Design review of the part built by this model. Coordinates are the model's own, in mm. A direction names the side the tool comes from. Give positions to 0.01 mm unless a question says otherwise; leave off trailing zeros. Order: outer loops, then holes, each group sorted by start corner. A loop starts at its lowest first (then second) coordinate and runs counter-clockwise, first axis right, second up. Notation, with made-up numbers: (4, 50) -> (25, 50) arc R28 cw to (25, 81) -> close; hole circle Ø5 at (-39.5, -18.5). An arc over 180 degrees is marked (long way). One line per item, written item: value. Start each with the question number.
1) Consider section C-C (x = -14.5). State the section outline as (y, z) points (3 decimals).
2) The part is to be moulded in two halves that separate along X. For faces 4 (the face through (-34.52, 8.1, 1.61)), 5 (the face through (-15, 0, 2)), 6 (the face through (-35.4, 16.3, 1.6)), say which applies: released by +X, released by -X, zero draft, split by the parting line, or undercut.
3) Consider section A-A (y = 10.75). State the section outline as (x, z) points (3 decimals).
4) Tool access review of faces 1 (the face through (-11.882, 14.445, 3.551)), 2 (the face through (-11.8, 16.1, 3.6)), 3 (the face through (-11.886, 1.745, 3.551)): name each direction out of +Z, -Z, +X, -X, +Y, -Y from which nothing blocks a thin tool from reaching the whole face with its end or side.
5) For pin 1 (0.8 mm diameter, centred on x = -22.5, z = 3.5, fed in from +Y); pin 2 (1.5 mm diameter, centred on x = -32.5, z = 3, fed in from +Y); pin 3 (8 mm diameter, centred on x = -32.5, y = 7.5, fed in from +Z) (3 decimals), all flat-tipped, find the tip position at first contact; note any pin that passes through.
6) Consider section B-B (z = 2.6). State the section outline as (x, y) points (3 decimals).
7) Wall thickness on line 1 along Y through (x, z) = (-20, 3.5); line 2 along Z through (x, y) = (-25, 8.25) (3 decimals); line 3 along X through (y, z) = (9, 0.4): over which ranges is each line inside the solid? List them lowest first. Write a range as from..to.
from build123d import *

# Parameters (mm, degrees)
F0_W     = 38.1
F0_H     = 19.05
F1_DEPTH = 3.175
F2_R     = 2.3454703993
F3_DEPTH = 3.176
F5_DEPTH = 0.762


with BuildPart() as f1:
    # F0 (on Top) → F1 (new body)
    with BuildSketch(Plane.XY):
        with Locations((-19.05, 9.525)):
            Rectangle(F0_W, F0_H)
    extrude(amount=F1_DEPTH)

    # F2 (on face) → F3 (cut, through all)
    with BuildSketch(Plane.XY.offset(3.175)):
        with Locations((-32.6583981514, 9.525)):
            Circle(F2_R)
        with BuildLine():
            ThreePointArc((-38.1, 9.9683756083), (-35.308362686, 16.3938160997), (-28.8257542998, 19.05))
            Line((-28.8257542998, 19.05), (-38.1, 19.05))
            Line((-38.1, 19.05), (-38.1, 9.9683756083))
        make_face()
        with BuildLine():
            ThreePointArc((-28.8257542998, 0), (-35.308362686, 2.6561839003), (-38.1, 9.0816243917))
            Line((-38.1, 9.0816243917), (-38.1, 0))
            Line((-38.1, 0), (-28.8257542998, 0))
        make_face()
    extrude(amount=-F3_DEPTH, mode=Mode.SUBTRACT)

    # F4 (on face) → F5 (join)
    with BuildSketch(Plane.XY.offset(3.175)):
        with BuildLine():
            add(Edge.make_bspline(
                [(-26.5377387404, 15.9110687673), (-26.7108747115, 15.8254740139), (-26.8840106825, 15.7398792605), (-27.0571466535, 15.654284507)],
                knots=[0, 0, 0, 0, 0.579415858, 0.579415858, 0.579415858, 0.579415858], degree=3))
            Line((-27.0571466535, 15.654284507), (-27.0571466535, 2.7385666035))
            add(Edge.make_bspline(
                [(-27.0571466535, 2.7385666035), (-27.0795693358, 2.6088543631), (-27.1225207817, 2.3603859501), (-26.8266557283, 2.183014384), (-26.6604257883, 2.1276841688), (-26.579702273, 2.1008150652)],
                knots=[0, 0, 0, 0, 0.359730405, 0.6890763936, 1, 1, 1, 1], degree=3))
            Line((-26.579702273, 2.1008150652), (-24.8697847128, 2.1008150652))
            add(Edge.make_bspline(
                [(-24.8697847128, 2.1008150652), (-24.8535585114, 1.9993606342), (-24.820613422, 1.7933712454), (-25.0545304604, 1.6052521128), (-25.323348361, 1.3860952125), (-24.5846096398, 1.4667534331), (-23.7811649583, 1.5054977354), (-22.5648546478, 1.5317740605), (-21.8525212711, 1.4849440744), (-20.7065855211, 1.6821403738), (-19.5728440966, 2.0528020227), (-19.1090591627, 2.3669456633), (-18.9018342644, 2.5073089637)],
                knots=[0, 0, 0, 0, 0.0654142898, 0.1328147962, 0.1852280569, 0.2717986293, 0.3900220534, 0.5225934237, 0.6267763583, 0.7573014589, 0.891559262, 1, 1, 1, 1], degree=3))
            Line((-18.9018342644, 2.5073089637), (-17.4452550709, 2.5073089637))
            add(Edge.make_bspline(
                [(-17.4452550709, 2.5073089637), (-17.416342407, 2.3859721487), (-17.3563210578, 2.1340825495), (-17.0722687387, 2.1058012821), (-16.9250462204, 2.0911432803)],
                knots=[0, 0, 0, 0, 0.4817063324, 1, 1, 1, 1], degree=3))
            Line((-16.9250462204, 2.0911432803), (-14.0298530459, 2.0911432803))
            Line((-14.0298530459, 2.0911432803), (-14.0298530459, 1.0200680699))
            Line((-14.0298530459, 1.0200680699), (-9.6812043339, 2.4914150126))
            add(Edge.make_bspline(
                [(-9.6812043339, 2.4914150126), (-9.6409541279, 2.4226709942), (-9.5613256349, 2.2866721227), (-9.3732923035, 2.143877022), (-9.146753539, 2.1258439034), (-8.9577295904, 2.2565656827), (-8.9125275808, 2.4112662698), (-8.8891088963, 2.4914150126)],
                knots=[0, 0, 0, 0, 0.2053847319, 0.4063203233, 0.6002825129, 0.7929105851, 1, 1, 1, 1], degree=3))
            Line((-8.8891088963, 2.4914150126), (-8.0058202147, 2.4914150126))
            Line((-8.0058202147, 2.4914150126), (-8.0058202147, 2.6511875913))
            Line((-8.0058202147, 2.6511875913), (-8.8891088963, 2.6511875913))
            add(Edge.make_bspline(
                [(-8.8891088963, 2.6511875913), (-8.9310142556, 2.7313268058), (-9.0111442626, 2.8845662941), (-9.2288589733, 2.9502078721), (-9.4263111029, 2.954461386), (-9.5681762791, 2.7983408667), (-9.6258537843, 2.6991547711), (-9.6537470818, 2.6511875913)],
                knots=[0, 0, 0, 0, 0.2243735688, 0.4290395288, 0.619806208, 0.816135277, 1, 1, 1, 1], degree=3))
            Line((-9.6537470818, 2.6511875913), (-13.9779066667, 4.1145463474))
            Line((-13.9779066667, 4.1145463474), (-13.9779066667, 3.2444412354))
            Line((-13.9779066667, 3.2444412354), (-16.2190869451, 3.2444412354))
            Line((-16.2190869451, 3.2444412354), (-16.2190869451, 8.471253328))
            Line((-16.2190869451, 8.471253328), (-12.8844231367, 8.471253328))
            add(Edge.make_bspline(
                [(-12.8844231367, 8.471253328), (-12.4868405129, 8.3912644099), (-11.73186638, 8.2393725502), (-10.9755685718, 7.6600087014), (-10.0278228964, 7.0776029449), (-9.2641156682, 6.3657609783), (-8.4323489729, 5.5191632424), (-8.2256469446, 5.2628506515), (-8.4263613819, 4.9657352945), (-8.4045845677, 4.387056325), (-8.3245215623, 3.8946895211), (-7.8349969225, 3.3357865397), (-7.3142777062, 2.8825893477), (-7.0247473195, 2.6306025684)],
                knots=[0, 0, 0, 0, 0.1119269029, 0.2125392595, 0.3204849305, 0.4302536688, 0.542538281, 0.5958954746, 0.6528186178, 0.7312491143, 0.8038353409, 0.8909284931, 1, 1, 1, 1], degree=3))
            Line((-7.0247473195, 2.6306025684), (-6.4539997838, 3.1442753971))
            Line((-6.4539997838, 3.1442753971), (-5.8452025987, 2.6306025684))
            add(Edge.make_bspline(
                [(-5.8452025987, 2.6306025684), (-5.7510163843, 2.5382953385), (-5.5793479133, 2.3700515982), (-5.3068982698, 2.3599422662), (-5.0234062685, 2.629445519), (-5.1548387797, 2.7849198566), (-5.217380356, 2.8589016292)],
                knots=[0, 0, 0, 0, 0.2794125753, 0.5092712331, 0.7664888973, 1, 1, 1, 1], degree=3))
            Line((-5.217380356, 2.8589016292), (-5.9783770703, 3.4867241047))
            Line((-5.9783770703, 3.4867241047), (-5.217380356, 4.190646112))
            Line((-5.217380356, 4.190646112), (-4.3422332965, 3.5247737542))
            add(Edge.make_bspline(
                [(-4.3422332965, 3.5247737542), (-4.2753552319, 3.4833438946), (-4.1355489457, 3.396736203), (-3.8719087651, 3.5821675688), (-3.8873582518, 3.8259382225), (-3.9635831277, 3.9291369105), (-4.0002227761, 3.9787422866)],
                knots=[0, 0, 0, 0, 0.2503847052, 0.5234205857, 0.7709185888, 1, 1, 1, 1], degree=3))
            Line((-4.0002227761, 3.9787422866), (-4.7757523134, 4.6124062501))
            Line((-4.7757523134, 4.6124062501), (-4.2272070423, 5.1231207326))
            Line((-4.2272070423, 5.1231207326), (-5.0594825298, 5.8891922235))
            add(Edge.make_bspline(
                [(-5.0594825298, 5.8891922235), (-5.2342245953, 6.0119831219), (-5.5535406301, 6.2363658579), (-5.9633037959, 6.3380845337), (-6.4624834448, 6.3629289512), (-6.9588518276, 6.326635918), (-7.2564382113, 6.1799434156), (-7.404985372, 6.1067184433)],
                knots=[0, 0, 0, 0, 0.2203014043, 0.4025691847, 0.6016033984, 0.8011310759, 1, 1, 1, 1], degree=3))
            add(Edge.make_bspline(
                [(-7.404985372, 6.1067184433), (-7.8012870357, 6.5100044394), (-8.5207565636, 7.2421975688), (-9.3143752369, 7.9809513855), (-10.4526059497, 8.667475744), (-11.8318533209, 9.304087771), (-13.1655398172, 9.6100287611), (-13.4780210852, 9.655550231), (-13.5454072432, 9.665475678)],
                knots=[0, 0, 0, 0, 0.1949094928, 0.3542547898, 0.528809926, 0.7243716486, 0.9083314981, 0.9676026394, 0.9676026394, 0.9676026394, 0.9676026394], degree=3))
            Line((-13.5454072432, 9.665475678), (-13.5536914822, 9.665475678))
            Line((-13.5536914822, 9.665475678), (-16.2297561765, 9.665475678))
            Line((-16.2297561765, 9.665475678), (-16.2297561765, 14.7121604532))
            Line((-16.2297561765, 14.7121604532), (-14.0407746658, 14.7121604532))
            Line((-14.0407746658, 14.7121604532), (-14.0407746658, 13.74643296))
            Line((-14.0407746658, 13.74643296), (-9.6628116444, 15.162833035))
            add(Edge.make_bspline(
                [(-9.6628116444, 15.162833035), (-9.5994792917, 15.0419453644), (-9.4666485777, 14.7884096682), (-8.9151551249, 14.924804863), (-8.8862007543, 15.0941198994), (-8.8744670414, 15.162833035)],
                knots=[0, 0, 0, 0, 0.3512906634, 0.7367442472, 1, 1, 1, 1], degree=3))
            Line((-8.8744670414, 15.162833035), (-8.0032702535, 15.162833035))
            Line((-8.0032702535, 15.162833035), (-8.0032702535, 15.3721110607))
            Line((-8.0032702535, 15.3721110607), (-8.8744670414, 15.3721110607))
            add(Edge.make_bspline(
                [(-8.8744670414, 15.3721110607), (-8.9258811293, 15.4535897314), (-9.0257330431, 15.6112970859), (-9.2823856435, 15.7082360182), (-9.5546444314, 15.5282819888), (-9.6134472425, 15.4120218853), (-9.6300745245, 15.3725532584)],
                knots=[0, 0, 0, 0, 0.2589067963, 0.4997338796, 0.7803818448, 0.9274568815, 0.9274568815, 0.9274568815, 0.9274568815], degree=3))
            Line((-9.6300745245, 15.3725532584), (-13.9726913457, 16.8323148205))
            Line((-13.9726913457, 16.8323148205), (-13.9726913457, 15.9259032621))
            Line((-13.9726913457, 15.9259032621), (-17.0669947674, 15.9259032621))
            add(Edge.make_bspline(
                [(-17.0669947674, 15.9259032621), (-17.2379265625, 15.8260077216), (-17.5305453526, 15.6574083814), (-17.5131075408, 15.4495405967), (-17.506107688, 15.3641048819)],
                knots=[0, 0, 0, 0, 0.5880208056, 1, 1, 1, 1], degree=3))
            Line((-17.506107688, 15.3641048819), (-18.9438629895, 15.3641048819))
            add(Edge.make_bspline(
                [(-18.9438629895, 15.3641048819), (-19.0730076064, 15.5122124042), (-19.3699914184, 15.8528037322), (-20.4455895706, 16.0592715534), (-21.1153456714, 16.3460981975), (-21.8142141514, 16.3983614206), (-22.1944451332, 16.4267960936)],
                knots=[0, 0, 0, 0, 0.212159, 0.4878855201, 0.7213756277, 1, 1, 1, 1], degree=3))
            Line((-22.1944451332, 16.4267960936), (-25.1324698329, 16.4267960936))
            add(Edge.make_bspline(
                [(-25.1324698329, 16.4267960936), (-25.0155507598, 16.3238609839), (-24.815014757, 16.1473098455), (-24.822982641, 15.9805868028), (-24.8263049871, 15.9110687673)],
                knots=[0, 0, 0, 0, 0.583032829, 1, 1, 1, 1], degree=3))
            Line((-24.8263049871, 15.9110687673), (-26.5377387404, 15.9110687673))
        make_face()
        with BuildLine():
            Line((-25.8164200932, 3.2712235115), (-25.8011277765, 8.5837785155))
            Line((-25.8011277765, 8.5837785155), (-17.506107688, 8.5837785155))
            Line((-17.506107688, 8.5837785155), (-17.4452550709, 3.1483727507))
            Line((-17.4452550709, 3.1483727507), (-17.4452550709, 2.7118595317))
            Line((-17.4452550709, 2.7118595317), (-18.8643243164, 2.7118595317))
            add(Edge.make_bspline(
                [(-18.8643243164, 2.7118595317), (-19.0815269134, 2.85521998), (-19.5524918726, 3.166071455), (-20.5984014649, 3.5593135264), (-21.5481955341, 3.753304769), (-22.1358927762, 3.7784602355), (-22.4202815443, 3.7906330545)],
                knots=[0, 0, 0, 0, 0.2329927864, 0.5052031588, 0.7605660635, 1, 1, 1, 1], degree=3))
            Line((-22.4202815443, 3.7906330545), (-25.1571703702, 3.7906330545))
            add(Edge.make_bspline(
                [(-25.1571703702, 3.7906330545), (-25.0642022591, 3.6982952356), (-24.8942335308, 3.5294788374), (-24.855211218, 3.3517428953), (-24.837533012, 3.2712235115)],
                knots=[0, 0, 0, 0, 0.5469718577, 1, 1, 1, 1], degree=3))
            Line((-24.837533012, 3.2712235115), (-25.8164200932, 3.2712235115))
        make_face(mode=Mode.SUBTRACT)
        with BuildLine():
            Line((-18.9293026924, 15.1415970176), (-17.506107688, 15.1415970176))
            Line((-17.506107688, 15.1415970176), (-17.428284511, 9.7119892016))
            Line((-17.428284511, 9.7119892016), (-25.822866708, 9.7119892016))
            Line((-25.822866708, 9.7119892016), (-25.822866708, 14.6800291177))
            Line((-25.822866708, 14.6800291177), (-24.7983376545, 14.6800291177))
            add(Edge.make_bspline(
                [(-25.1186843961, 14.1409179196), (-25.0576893253, 14.2285084067), (-24.9435954911, 14.3923500806), (-24.7955780658, 14.5766326071), (-24.7956461395, 14.6560214032), (-24.7983376545, 14.6800291177)],
                knots=[0, 0, 0, 0, 0.4063243511, 0.7600467132, 0.9204385352, 0.9204385352, 0.9204385352, 0.9204385352], degree=3))
            Line((-25.1186843961, 14.1409179196), (-21.7460282147, 14.1409179196))
            add(Edge.make_bspline(
                [(-18.9293026924, 15.1415970176), (-19.0907602148, 15.0203952413), (-19.4210171313, 14.772480345), (-20.0535811337, 14.5777947582), (-20.8713014134, 14.222314871), (-21.4546989083, 14.168027318), (-21.7460282147, 14.1409179196)],
                knots=[0, 0, 0, 0, 0.2237759252, 0.4577274938, 0.7292071452, 1, 1, 1, 1], degree=3))
        make_face(mode=Mode.SUBTRACT)
    extrude(amount=F5_DEPTH)


solid = f1.part
Checked values:
1. outline: (0, 0) -> (19.05, 0) -> (19.05, 3.175) -> (15.926, 3.175) -> (15.926, 3.937) -> (14.712, 3.937) -> (14.712, 3.175) -> (9.665, 3.175) -> (9.665, 3.937) -> (8.471, 3.937) -> (8.471, 3.175) -> (3.244, 3.175) -> (3.244, 3.937) -> (2.091, 3.937) -> (2.091, 3.175) -> (0, 3.175) -> close
2. face 4: undercut
2. face 5: zero draft
2. face 6: released by -X
3. outline: (-38.048, 0) -> (-34.659, 0) -> (-34.659, 3.175) -> (-38.048, 3.175) -> close; (-30.658, 0) -> (0, 0) -> (0, 3.175) -> (-16.23, 3.175) -> (-16.23, 3.937) -> (-17.443, 3.937) -> (-17.443, 3.175) -> (-25.823, 3.175) -> (-25.823, 3.937) -> (-27.057, 3.937) -> (-27.057, 3.175) -> (-30.658, 3.175) -> close
4. face 1: +Z
4. face 2: +Z, +Y
4. face 3: +Z, -Y
5. pin 1: stops at y = 19.05
5. pin 2: stops at y = 18.57
5. pin 3: stops at z = 3.175
6. outline: (-38.1, 9.082) arc R9.303 ccw to (-28.826, 0) -> (0, 0) -> (0, 19.05) -> (-28.826, 19.05) arc R9.303 ccw to (-38.1, 9.968) -> close; hole circle Ø4.691 at (-32.658, 9.525)
7. line 1: y = 1.93..3.32, 8.58..9.71, 14.58..15.97
7. line 2: z = 0..3.175
7. line 3: x = -38.1..-34.94, -30.37..0
